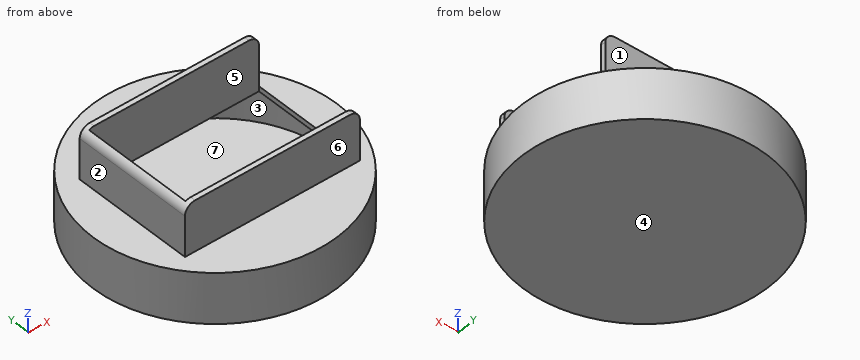
```python
from build123d import *

# Parameters (mm, degrees)
F0_R        = 61.5660175878
F1_DEPTH    = 25.4
F2_W        = 88.528262917
F2_H        = 61.6074204445
F3_DEPTH    = 25.4
F4_T        = 2.54
F4_T3_DEPTH = 93.608262917
F4_T5_DEPTH = 66.6874204445
F5_T1_DEPTH = 87.0074204445
F6_R        = 5.08


# Not quite as in the source:
# - a fillet or chamfer that OpenCascade refuses, or shapes differently, is made with other operations: its cross-section is extruded or revolved along the edge and cut away or added
# - a shell that OpenCascade refuses in one call is made with other operations: the cavity is built on its own and cut out


with BuildPart() as f1:
    # F0 (on Top) → F1 (new body)
    with BuildSketch(Plane.XY):
        with Locations((-52.3894988, 0)):
            Circle(F0_R)
    extrude(amount=F1_DEPTH)

    # F2 (on face) → F3 (join)
    with BuildSketch(Plane.XY.offset(25.4)):
        with Locations((-50.8173767012, -0.9788312018)):
            Rectangle(F2_W, F2_H)
    extrude(amount=F3_DEPTH)

    # F4: shell of thickness 2.54, made by hand


with BuildPart() as f4_core1:
    # F4_t2: copy of F1
    add(f1.part)

    # the walls: a layer under each face that stays
    f4_faces = [f4_core1.faces().sort_by_distance(p)[0] for p in [
        (-113.9555163879, 0, 12.7),
        (-52.3894988, 0, 0),
        (-93.4335105253, -41.0440117252, 25.4),
        (-50.8173767012, 29.8248790205, 38.1),
        (-95.0815081596, -0.9788312018, 38.1),
        (-50.8173767012, -31.782541424, 38.1),
    ]]
    thicken(f4_faces, amount=-F4_T, mode=Mode.SUBTRACT)

    # F4_s4 → F4_t3 (cut)
    with BuildSketch(Plane.YZ.offset(-97.6215081596)):
        Polygon((29.8502790205, 25.4254), (29.8248790205, 22.86), (27.2848790205, 22.86), (27.2848790205, 25.4), align=None)
        Polygon((-31.807941424, 25.4254), (-31.782541424, 22.86), (-29.242541424, 22.86), (-29.242541424, 25.4), align=None)
    extrude(amount=F4_T3_DEPTH, mode=Mode.SUBTRACT)

    # F4_s6 → F4_t5 (cut)
    with BuildSketch(Plane.XZ.offset(-32.3648790205)):
        Polygon((-95.1069081596, 25.4254), (-95.0815081596, 22.86), (-92.5415081596, 22.86), (-92.5415081596, 25.4), align=None)
    extrude(amount=F4_T5_DEPTH, mode=Mode.SUBTRACT)


with BuildPart() as f1_1:
    add(f1.part)

    # what is left inside the walls is the cavity
    f4_cavity = [f4_core1.part.solids().sort_by_distance(p)[0] for p in [
        (-52.389499, -19.675339, 2.5654),
    ]]
    add(f4_cavity, mode=Mode.SUBTRACT)

    # F5: fillet of radius 5.08 on 1 edges, made by hand

    # F5_s2 → F5_t1 (cut)
    with BuildSketch(Plane.XZ.offset(-42.5248790205)):
        with BuildLine():
            ThreePointArc((-95.0815081596, 45.72), (-93.5936106081, 49.3121024484), (-90.0015081596, 50.8))
            Line((-90.0015081596, 50.8), (-95.0815081596, 50.8))
            Line((-95.0815081596, 50.8), (-95.0815081596, 45.72))
        make_face()
    extrude(amount=F5_T1_DEPTH, mode=Mode.SUBTRACT)

    # F6
    f6_edges = [f1_1.edges().sort_by_distance(p)[0] for p in [
        (-6.553245, -30.512541, 50.8),
        (-6.553245, 28.554879, 50.8),
    ]]
    fillet(f6_edges, radius=F6_R)


solid = f1_1.part
```
Work out the finished part from the listing and answer in its coordinate system (mm). Face numbers are marked on the shaded views. A direction names the side the tool comes from. Round coordinates to 2 decimals unless told otherwise and drop trailing zeros. Write each loop counter-clockwise with the first axis right and the second up, starting at its lowest first coordinate (ties: lowest second). Pieces come first, ordered by that corner, then holes. Notation, with made-up numbers: (59, 3) - (109, 3) arc R15 cw to (109, 13) - close; hole circle Ø5 at (-2, -35.5). An arc over 180 degrees is marked (long way). Return JSON: item names as keys, results as strings. Group by question number.
Q1. The part is cut by section D-D on z = 18.5. Write down the section's boundary in (x, y).
Q2. Each of these flat-tipped pins is pushed along its axis until it touches: pin 1 Ø8.5 at (x, z) = (-69, 38) entering from -Y; pin 2 Ø5 at (x, y) = (-34, 33) entering from +Z; pin 3 Ø12.5 at (x, z) = (-51.5, 40) entering from +Y. Where does it stop, or does it pass through?
Q3. The part is cut by section B-B on z = 41. Write down the section's boundary in (x, y), then the cut area to 3 significant figures.
Q4. The part is cut by section C-C on x = -99.5. Write down the section's boundary in (y, z), then the cut area to 3 significant figures.
Q5. For the marked faces 1, 2 and 3, determine the directions among +Z, -Z, +X, -X, +Y, -Y from which every point of the face is accessible in a straight line to the end or side of a thin tool.
Q6. The part is cut by section A-A on y = 0. Write down the section's boundary in (x, z), then the cut area to 3 significant figures.
Q7. Find the intervals of material crossed by L1, parallel to Z at x = -70.5, y = -33.5; L2, parallel to Y at x = -77, z = 34.5; L3, parallel to X at y = 23, z = 25.5, in increasing order.
Q8. The mould has two halves that part along Y. Classify the marked faces 4, 5, 6 and 7: released by +Y, released by -Y, zero draft, split by the parting line, or undercut.
Solved:
{
 "1": {"outline": "circle Ø123.13 at (-52.39, 0); hole circle Ø118.05 at (-52.39, 0)"},
 "2": {"pin 1": "y = -31.78", "pin 2": "z = 25.4", "pin 3": "y = 29.82"},
 "3": {"outline": "(-95.08, -31.78) - (-6.55, -31.78) - (-6.55, -29.24) - (-92.54, -29.24) - (-92.54, 27.28) - (-6.55, 27.28) - (-6.55, 29.82) - (-95.08, 29.82) - close", "area": "593 mm²"},
 "4": {"outline": "(-39.64, 0) - (39.64, 0) - (39.64, 25.4) - (-39.64, 25.4) - close; hole (-35.56, 2.54) - (35.56, 2.54) - (35.56, 22.86) - (-35.56, 22.86) - close", "area": "568 mm²"},
 "5": {"face 1": "+Z, +X, -X, +Y", "face 2": "+Z, -X, +Y, -Y", "face 3": "none"},
 "6": {"outline": "(-113.96, 0) - (9.18, 0) - (9.18, 25.4) - (-6.55, 25.4) - (-6.55, 22.86) - (6.64, 22.86) - (6.64, 2.54) - (-111.42, 2.54) - (-111.42, 22.86) - (-92.54, 22.86) - (-92.54, 50.12) arc R5.08 ccw to (-95.08, 45.72) - (-95.08, 25.4) - (-113.96, 25.4) - close", "area": "570 mm²"},
 "7": {"L1": "0 to 2.54, 22.86 to 25.4", "L2": "-31.78 to -29.24, 27.28 to 29.82", "L3": "-95.08 to -92.54"},
 "8": {"face 4": "zero draft", "face 5": "undercut", "face 6": "released by -Y", "face 7": "undercut"}
}
